The listing builds one solid part. Answer for the finished solid, in the listing's coordinates (mm). Give positions to 0.01 mm unless a question says otherwise; leave off trailing zeros. Write each loop counter-clockwise with the first axis right and the second up, starting at its lowest first coordinate (ties: lowest second). Pieces come first, ordered by that corner, then holes. Notation, with made-up numbers: (85.5, -21) -> (119.5, -21) arc R18 cw to (119.5, 6) -> close; hole circle Ø10 at (65, 74). An arc over 180 degrees is marked (long way). Put each result on its own line as item: value. Start each with the question number.
1) A cutting plane is placed at B-B (z = -10.5). Write down the section's boundary in (x, y), then the cut area to 3 significant figures.
2) For a pull along Z with two mould halves and no side action, classify faces 1 (the flat face through (-1, 3, -1)), 2 (the cylindrical face through (72.143, 1.521, -31.347)) as released by +Z, released by -Z, zero draft, split by the parting line, or undercut.
3) A flat-ended cylindrical pin translates along its axis: pin 1 Ø3 at (x, z) = (58.495, -31) entering from +Y. Find the tip coordinate at first contact, or state that the pin passes through.
4) A cutting plane is placed at A-A (x = -87.5). Write down the section's boundary in (y, z), then the cut area to 3 significant figures.
5) A cutting plane is placed at C-C (y = 0.65). Give the number of separate pieces and of enclosed holes in the cut face, then the cut area to 3 significant figures.
6) Find the intervals of material crossed by line 1 along X through (y, z) = (2.65, 21.5); line 2 along X through (y, z) = (1.35, -20.5); line 3 along X through (y, z) = (2, -31) (3 decimals), in increasing order. Write a range as from..to.
from build123d import *

# Parameters (mm, degrees)
SKETCH1_W           = 190
SKETCH1_H           = 80
BOSS_EXTRUDE1_DEPTH = 3
SKETCH4_R           = 1.4
SKETCH4_R_2         = 1.6
CUT_EXTRUDE2_DEPTH  = 3


with BuildPart() as part:
    # Sketch1 → Boss-Extrude1 (new body)
    with BuildSketch(Plane(origin=(0, 0, 0), x_dir=(1, 0, 0), z_dir=(0, 1, 0))):
        Rectangle(SKETCH1_W, SKETCH1_H)
        with BuildLine():
            Line((-90, 6.5), (-90, 31.5))
            ThreePointArc((-90, 31.5), (-87.5, 34), (-85, 31.5))
            Line((-85, 31.5), (-85, 6.5))
            ThreePointArc((-85, 6.5), (-87.5, 4), (-90, 6.5))
        make_face(mode=Mode.SUBTRACT)
        with BuildLine():
            Line((-90, -6.5), (-90, -31.5))
            ThreePointArc((-90, -31.5), (-87.5, -34), (-85, -31.5))
            Line((-85, -31.5), (-85, -6.5))
            ThreePointArc((-85, -6.5), (-87.5, -4), (-90, -6.5))
        make_face(mode=Mode.SUBTRACT)
        with BuildLine():
            Line((90, 6.5), (90, 31.5))
            ThreePointArc((90, 31.5), (87.5, 34), (85, 31.5))
            Line((85, 31.5), (85, 6.5))
            ThreePointArc((85, 6.5), (87.5, 4), (90, 6.5))
        make_face(mode=Mode.SUBTRACT)
        with BuildLine():
            Line((90, -6.5), (90, -31.5))
            ThreePointArc((90, -31.5), (87.5, -34), (85, -31.5))
            Line((85, -31.5), (85, -6.5))
            ThreePointArc((85, -6.5), (87.5, -4), (90, -6.5))
        make_face(mode=Mode.SUBTRACT)
    extrude(amount=BOSS_EXTRUDE1_DEPTH)

    # Sketch4 → Cut-Extrude2 (cut)
    with BuildSketch(Plane(origin=(0, 3, 0), x_dir=(1, 0, 0), z_dir=(0, 1, 0))):
        with Locations(Location((56.1, 20.5, 0), (0, 0, 270))):
            Circle(SKETCH4_R)
        with Locations(Location((76.1, 20.5, 0), (0, 0, 270))):
            Circle(SKETCH4_R)
        with Locations(Location((58.495, 31, 0), (0, 0, 270))):
            Circle(SKETCH4_R_2)
        with Locations(Location((73.705, 31, 0), (0, 0, 270))):
            Circle(SKETCH4_R_2)
    extrude(amount=-CUT_EXTRUDE2_DEPTH, mode=Mode.SUBTRACT)


solid = part.part
Reply:
1. outline: (-95, 0) -> (-90, 0) -> (-90, 3) -> (-95, 3) -> close; (-85, 0) -> (85, 0) -> (85, 3) -> (-85, 3) -> close; (90, 0) -> (95, 0) -> (95, 3) -> (90, 3) -> close
1. area: 540 mm2
2. face 1: zero draft
2. face 2: undercut
3. pin 1: passes through
4. outline: (0, -40) -> (3, -40) -> (3, -34) -> (0, -34) -> close; (0, -4) -> (3, -4) -> (3, 4) -> (0, 4) -> close; (0, 34) -> (3, 34) -> (3, 40) -> (0, 40) -> close
4. area: 60.0 mm2
5. separate pieces: 1
5. enclosed holes: 8
5. area: 14,600 mm2
6. line 1: x = -95..-90, -85..85, 90..95
6. line 2: x = -95..-90, -85..54.7, 57.5..74.7, 77.5..85, 90..95
6. line 3: x = -95..-90, -85..56.895, 60.095..72.105, 75.305..85, 90..95
